Job drawing, mm, ordinate dimensions from the low corner. One solid piece. A direction names the side the tool comes from. Give positions to 0.01 mm unless a question says otherwise; leave off trailing zeros. Loops run counter-clockwise (first coordinate to the right, second up) from the corner with the lowest first, then second, coordinate; pieces in that order, holes last. Notation, with made-up numbers: M -31.5,16.25 L 25.5,16.25 A19 cw 25.5,40.25 Z; hole C -27,-5.5 d4. An arc over 180 degrees is marked long. Answer as CSV lines item,"result".
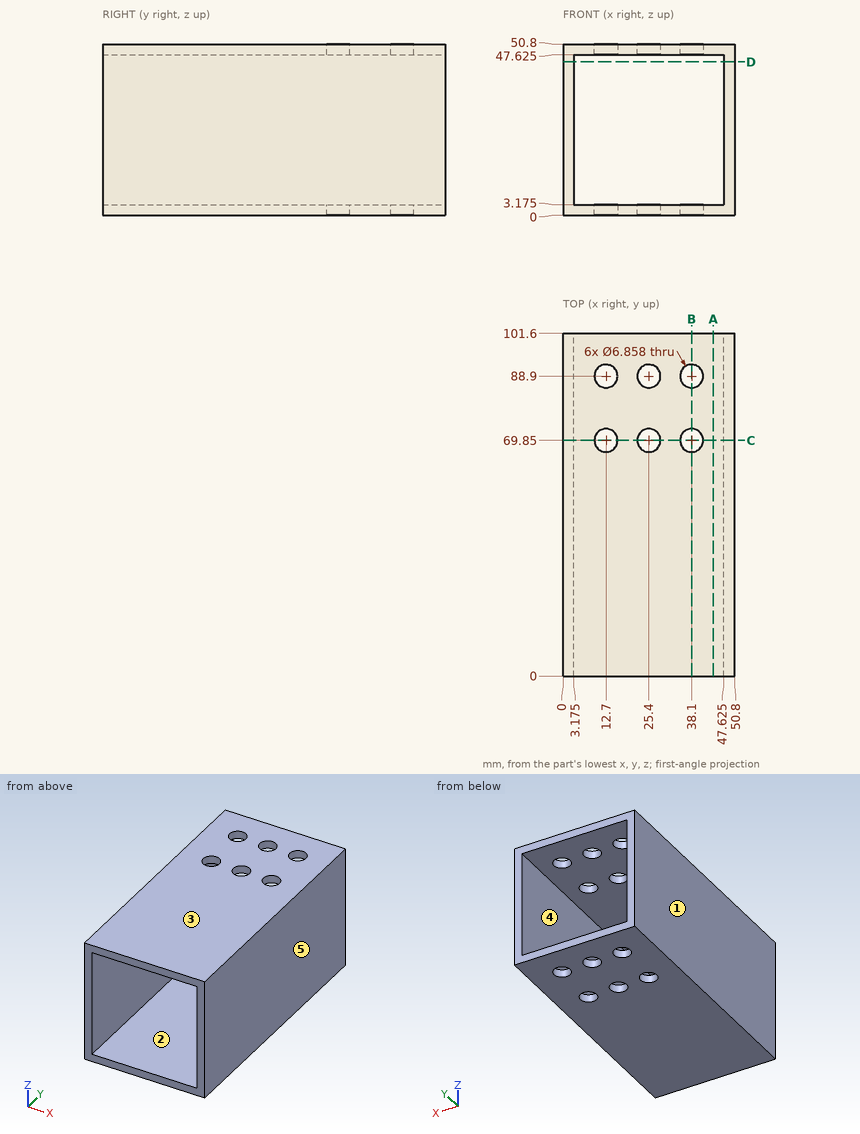
1) Band-saw the part on A-A on x = 44.5. Give the cut face in (y, z) (3 decimals).
Answer below:
outline,"M 0,0 L 101.6,0 L 101.6,3.175 L 0,3.175 Z; M 0,47.625 L 101.6,47.625 L 101.6,50.8 L 0,50.8 Z"
2) Band-saw the part on D-D on z = 45.5. Give the cut face in (x, y) (3 decimals), and give its area (3 significant figures).
Answer below:
outline,"M 0,0 L 3.175,0 L 3.175,101.6 L 0,101.6 Z; M 47.625,0 L 50.8,0 L 50.8,101.6 L 47.625,101.6 Z"
area,"645 mm^2"
3) Flat gauge pins, fed straight in: pin 1 (4 mm diameter, centred on x = 25.4, y = 69.85, fed in from +Z); pin 2 (9 mm diameter, centred on x = 12.7, y = 88.9, fed in from +Z). Where does each tip first touch, or does it go through?
Answer below:
pin 1,"passes through"
pin 2,"stops at z = 50.8"
4) Band-saw the part on B-B on x = 38.1. Give the cut face in (y, z) (3 decimals), and give its area (3 significant figures).
Answer below:
outline,"M 0,0 L 66.421,0 L 66.421,3.175 L 0,3.175 Z; M 0,47.625 L 66.421,47.625 L 66.421,50.8 L 0,50.8 Z; M 73.279,0 L 85.471,0 L 85.471,3.175 L 73.279,3.175 Z; M 73.279,47.625 L 85.471,47.625 L 85.471,50.8 L 73.279,50.8 Z; M 92.329,0 L 101.6,0 L 101.6,3.175 L 92.329,3.175 Z; M 92.329,47.625 L 101.6,47.625 L 101.6,50.8 L 92.329,50.8 Z"
area,"558 mm^2"
5) Which spindle directions (+Z, -Z, +X, -X, +Y, -Y) get a long thin tool onto all of the face, cutting with end or side? Do the marked faces 4 and 5. Say none if no direction does.
Answer below:
face 4,"+Y, -Y"
face 5,"+Z, -Z, +X, +Y, -Y"
6) Mould opens along X. For the marked faces 1, 2 and 3 say: +X half, -X half, draft (parallel to the pull), parting line (faces both ways), or undercut.
Answer below:
face 1,"-X half"
face 2,"undercut"
face 3,"draft"
7) Band-saw the part on C-C on y = 69.85. Give the number of separate pieces and of enclosed holes in the cut face, and give its area (3 significant figures).
Answer below:
separate pieces,"6"
enclosed holes,"0"
area,"474 mm^2"
8) Drill centre lines: line 1 (X direction, y = 88.9, z = 0.7); line 2 (Y direction, x = 25.4, z = 50.1); line 3 (X direction, y = 84.5, z = 22.5) (3 decimals). Where is each one in solid material? Low to high. Write a range as from..to.
Answer below:
line 1,"x = 0..9.27, 16.13..21.97, 28.83..34.67, 41.53..50.8"
line 2,"y = 0..66.42, 73.28..85.47, 92.33..101.6"
line 3,"x = 0..3.175, 47.625..50.8"
